```python
from build123d import *

# Parameters (mm, degrees)
F0_R     = 10
F0_R_2   = 4.5
F1_DEPTH = 15
F2_SIZE  = 1.5
F3_SIZE  = 0.3


with BuildPart() as f1:
    # F0 (on Top) → F1 (new body)
    with BuildSketch(Plane.XY):
        Circle(F0_R)
        Circle(F0_R_2, mode=Mode.SUBTRACT)
    extrude(amount=-F1_DEPTH)

    # F2
    f2_edges = [f1.edges().sort_by_distance(p)[0] for p in [
        (-10, 0, 0),
    ]]
    chamfer(f2_edges, length=F2_SIZE)

    # F3
    f3_edges = [f1.edges().sort_by_distance(p)[0] for p in [
        (-4.5, 0, 0),
    ]]
    chamfer(f3_edges, length=F3_SIZE)


solid = f1.part
```
For this review, take the finished solid that the model builds, in its own axes (mm). Coordinates: 2 decimals unless noted, no trailing zeros. Loops run counter-clockwise (first coordinate to the right, second up) from the corner with the lowest first, then second, coordinate; pieces in that order, holes last. Notation, with made-up numbers: (79.25, 11) -> (84.25, 11) arc R26 cw to (84.25, 39) -> close; hole circle Ø10 at (38.5, 86.5). An arc over 180 degrees is marked (long way). Return JSON: item names as keys, results as strings. Group by question number.
(1) To check wall thickness, follow L1, parallel to Y at x = 0, z = -10.25; L2, parallel to Y at x = -2.75, z = -2.5; L3, parallel to X at y = 1.5, z = -5.5. State the ranges of each line that lie inside material, in increasing order.
(2) Mouldability with a two-part tool opening along Y and no side actions: class faces 1 (the flat face through (4.3, -2.1, -15)), 2 (the cylindrical face through (-2.17, -9.76, -8.16)), 3 (the cylindrical face through (-0.59, 4.46, -7.55)) as pulls with the +Y half, pulls with the -Y half, needs draft (parallel to the pull), parting line crosses it, or undercut.
(3) Consider section C-C, the plane z = -7. Give the boundary of the cut face in (x, y), plus the area to 3 significant figures.
(4) For pin 1 Ø3 at (x, z) = (-3.5, -4.5) entering from -Y; pin 2 Ø5 at (y, z) = (-8, -7.5) entering from +X; pin 3 Ø3 at (y, z) = (-6, -10.5) entering from -X, all flat-tipped, find the tip position at first contact; note any pin that passes through.
(5) Consider section A-A, the plane x = 0. Give the boundary of the cut face in (y, z).
Results below:
{
 "1": {"L1": "y = -10 to -4.5, 4.5 to 10", "L2": "y = -9.61 to -3.56, 3.56 to 9.61", "L3": "x = -9.89 to -4.24, 4.24 to 9.89"},
 "2": {"face 1": "needs draft", "face 2": "parting line crosses it", "face 3": "undercut"},
 "3": {"outline": "circle Ø20 at (0, 0); hole circle Ø9 at (0, 0)", "area": "251 mm2"},
 "4": {"pin 1": "stops at y = -9.8", "pin 2": "stops at x = 8.35", "pin 3": "stops at x = -8.93"},
 "5": {"outline": "(-10, -15) -> (-4.5, -15) -> (-4.5, -0.3) -> (-4.8, 0) -> (-8.5, 0) -> (-10, -1.5) -> close; (4.5, -15) -> (10, -15) -> (10, -1.5) -> (8.5, 0) -> (4.8, 0) -> (4.5, -0.3) -> close"}
}
